Verification items for the finished model (mm, model axes). A direction names the side the tool comes from. Coordinates: 2 decimals unless noted, no trailing zeros. Write each loop counter-clockwise with the first axis right and the second up, starting at its lowest first coordinate (ties: lowest second). Pieces come first, ordered by that corner, then holes. Notation, with made-up numbers: M 15,89.25 L 44,89.25 A21 ccw 44,120.25 Z; hole C -27.75,10.5 d9. An arc over 180 degrees is marked long. Answer in a Markdown table with one row per item.
from build123d import *

# Parameters (mm, degrees)
CAMBER_BLOCK_EXTRUDE_DEPTH                          = 50.8
CSK_FOR_1_4_FLAT_HEAD_MACHINE_SCREW_100_D           = 6.7564
CSK_FOR_1_4_FLAT_HEAD_MACHINE_SCREW_100_CSINK_D     = 13.4874
CSK_FOR_1_4_FLAT_HEAD_MACHINE_SCREW_100_CSINK_ANGLE = 82
CUT_EXTRUDE1_REACH                                  = 75.171
SKETCH5_R                                           = 4.7625


with BuildPart() as part:
    # Sketch1 → Camber Block Extrude (new body)
    with BuildSketch(Plane(origin=(0, 0, 0), x_dir=(1, 0, 0), z_dir=(0, 1, 0))):
        Polygon((0, 0), (42.015665571, 0), (42.015665571, 5.5499), (10.265665571, 5.5499), (10.265665571, 26.2001), (42.015665571, 26.2001), (42.015665571, 31.75), (0, 31.75), align=None)
    extrude(amount=CAMBER_BLOCK_EXTRUDE_DEPTH)

    # CSK for 1/4 Flat Head Machine Screw (100)1 (through all)
    with Locations(Plane(origin=(10.265665571, 0, 0), x_dir=(0, 0, -1), z_dir=(1, 0, 0))):
        with Locations((15.875, 12.7), (15.875, 38.1)):
            CounterSinkHole(CSK_FOR_1_4_FLAT_HEAD_MACHINE_SCREW_100_D / 2, CSK_FOR_1_4_FLAT_HEAD_MACHINE_SCREW_100_CSINK_D / 2, counter_sink_angle=CSK_FOR_1_4_FLAT_HEAD_MACHINE_SCREW_100_CSINK_ANGLE)

    # Cut-Extrude1: up to this face of the body (flat: up to its plane)
    cut_extrude1_end = Plane(part.part.faces().sort_by_distance((21.007832786, 25.4, -31.75))[0])
    # Sketch5 → Cut-Extrude1 (cut, up to the picked face)
    with BuildSketch(Plane.XY, mode=Mode.PRIVATE) as cut_extrude1_sk1:
        with Locations((29.315665571, 25.4)):
            Circle(SKETCH5_R)
    cut_extrude1_tool1 = split(extrude(cut_extrude1_sk1.sketch, amount=-CUT_EXTRUDE1_REACH, mode=Mode.PRIVATE), bisect_by=cut_extrude1_end, keep=Keep.BOTH, mode=Mode.PRIVATE)
    # Sketch5 → Cut-Extrude1 (cut, up to the picked face)
    with BuildSketch(Plane.XY, mode=Mode.PRIVATE) as cut_extrude1_sk2:
        with BuildLine():
            Line((0, 0), (33.881349019, 15.26875176))
            ThreePointArc((33.881349019, 15.26875176), (40.428165571, 25.4), (33.881349019, 35.53124824))
            Line((33.881349019, 35.53124824), (0, 50.8))
            Line((0, 50.8), (42.015665571, 50.8))
            Line((42.015665571, 50.8), (42.015665571, 0))
            Line((42.015665571, 0), (0, 0))
        make_face()
    cut_extrude1_tool2 = split(extrude(cut_extrude1_sk2.sketch, amount=-CUT_EXTRUDE1_REACH, mode=Mode.PRIVATE), bisect_by=cut_extrude1_end, keep=Keep.BOTH, mode=Mode.PRIVATE)
    add(cut_extrude1_tool1.solids().sort_by(Axis((29.315666, 25.4, 0), (0, 0, -1)))[0], mode=Mode.SUBTRACT)
    add(cut_extrude1_tool2.solids().sort_by(Axis((17.211529, 7.033349, 0), (0, 0, -1)))[0], mode=Mode.SUBTRACT)


solid = part.part
1) Sectioned sample at A-A (y = 25.4). Record the cut outline in (x, z).
Response values:
| item | result |
|---|---|
| outline | M 0,-31.75 L 24.55,-31.75 L 24.55,-26.2 L 10.27,-26.2 L 10.27,-5.55 L 24.55,-5.55 L 24.55,0 L 0,0 Z; M 34.08,-31.75 L 40.43,-31.75 L 40.43,-26.2 L 34.08,-26.2 Z; M 34.08,-5.55 L 40.43,-5.55 L 40.43,0 L 34.08,0 Z |
2) Depth check by flat-ended pin: pin 1 (10 mm diameter, centred on y = 20, z = -19, fed in from +X); pin 2 (4 mm diameter, centred on y = 38.1, z = -15.875, fed in from +X); pin 3 (5 mm diameter, centred on x = 6, z = -27.5, fed in from -Y). Enter the tip coordinate at first touch or a pass-through.
Response values:
| item | result |
|---|---|
| pin 1 | stops at x = 10.27 |
| pin 2 | passes through |
| pin 3 | stops at y = 1.58 |
3) Thickness scan on L1, parallel to Z at x = 1.5, y = 12.7; L2, parallel to Z at x = 35.5, y = 23; L3, parallel to X at y = 22, z = -23. Record the ranges inside material, lowest first. Write a range as [from, to].
Response values:
| item | result |
|---|---|
| L1 | z = [-31.75, -19.25], [-12.5, 0] |
| L2 | z = [-31.75, -26.2], [-5.55, 0] |
| L3 | x = [0, 10.27] |
4) Sectioned sample at B-B (x = 17.5). Record the cut outline in (y, z).
Response values:
| item | result |
|---|---|
| outline | M 7.89,-31.75 L 42.91,-31.75 L 42.91,-26.2 L 7.89,-26.2 Z; M 7.89,-5.55 L 42.91,-5.55 L 42.91,0 L 7.89,0 Z |
5) Sectioned sample at D-D (x = 29.5). Record the cut outline in (y, z).
Response values:
| item | result |
|---|---|
| outline | M 13.29,-31.75 L 20.64,-31.75 L 20.64,-26.2 L 13.29,-26.2 Z; M 13.29,-5.55 L 20.64,-5.55 L 20.64,0 L 13.29,0 Z; M 30.16,-31.75 L 37.51,-31.75 L 37.51,-26.2 L 30.16,-26.2 Z; M 30.16,-5.55 L 37.51,-5.55 L 37.51,0 L 30.16,0 Z |
6) Tool access check on faces 1 (the face through (0, 25, -16)), 2 (the face through (22, 25, -26.2)). Record the directions out of +Z, -Z, +X, -X, +Y, -Y that give a thin tool (end or side, any length) a straight path to the whole face; none if there is none.
Response values:
| item | result |
|---|---|
| face 1 | +Z, -Z, -X, +Y, -Y |
| face 2 | +X, +Y, -Y |
7) Release check for a two-part mould opening along Z. For faces 3 (the face through (15, 25, 0)), 4 (the face through (22, 25, -5.55)), 5 (the face through (9.65, 46.45, -15.65)), 6 (the face through (3.152, 11.406, -12.754)) record: +Z half, -Z half, draft (parallel to the pull), parting line (faces both ways), or undercut.
Response values:
| item | result |
|---|---|
| face 3 | +Z half |
| face 4 | undercut |
| face 5 | draft |
| face 6 | undercut |
8) Sectioned sample at C-C (y = 38.1). Record the cut outline in (x, z), then the cut area to 3 significant figures.
Response values:
| item | result |
|---|---|
| outline | M 0,-31.75 L 28.18,-31.75 L 28.18,-26.2 L 10.27,-26.2 L 10.27,-22.62 L 6.39,-19.25 L 0,-19.25 Z; M 0,-12.5 L 6.39,-12.5 L 10.27,-9.13 L 10.27,-5.55 L 28.18,-5.55 L 28.18,0 L 0,0 Z |
| area | 442 mm² |
